Verification items for the finished model (mm, model axes). A direction names the side the tool comes from. Give positions to 0.01 mm unless a question says otherwise; leave off trailing zeros. Write each loop counter-clockwise with the first axis right and the second up, starting at its lowest first coordinate (ties: lowest second). Pieces come first, ordered by that corner, then holes. Notation, with made-up numbers: (25, 81.5) -> (32, 81.5) arc R25 cw to (32, 97.5) -> close; hole circle Ø7 at (21, 72). An arc over 180 degrees is marked (long way). Answer as CSV lines item,"result". Start each with the question number.
1) Tool access check on faces 4 (the flat face through (43, 3, 7)), 5 (the flat face through (14, 12, 11)), 6 (the flat face through (50, 3, 3)), 7 (the flat face through (7, 14, 21)). Record the directions out of +Z, -Z, +X, -X, +Y, -Y that give a thin tool (end or side, any length) a straight path to the whole face; none if there is none.
2) Mould release check, pull along Z, two halves, no side actions. Record for faces 1 (the flat face through (19, 0, 14)), 2 (the flat face through (43, 3, 21)), 3 (the flat face through (19, 6, 28)): released by +Z, released by -Z, zero draft, split by the parting line, or undercut.
3) Material ranges on L1, parallel to Y at x = 19, z = 7.75; L2, parallel to Y at x = 7.5, z = 16.5, recorded low to high.
4) Sectioned sample at A-A on y = 4.75. Record the cut outline in (x, z).
5) Sectioned sample at C-C on x = 5. Record the cut outline in (y, z), and give its area (3 significant figures).
6) Gauge pin test, flat ends, axial feed: pin 1 Ø4 at (x, z) = (10.5, 22.5) entering from +Y; pin 2 Ø4 at (x, y) = (19, 9.5) entering from +Z; pin 3 Ø14 at (x, z) = (35, 8) entering from +Y; pin 4 Ø3.5 at (x, y) = (6.5, 18.5) entering from +Z. Record the tip position at first contact, or that the pin passes through.
7) Sectioned sample at B-B on z = 24.5. Record the cut outline in (x, y).
8) Sectioned sample at D-D on y = 10. Record the cut outline in (x, z).
```python
from build123d import *

# Parameters (mm, degrees)
EXTRUDE_1_DEPTH     = 28
SKETCH_2_W          = 14
SKETCH_2_H          = 14
CUT_EXTRUDE_1_DEPTH = 7
CUT_EXTRUDE_2_REACH = 23


with BuildPart() as part:
    # 스케치1 → 보스-돌출1 (new body)
    with BuildSketch(Plane.XY):
        Polygon((14, 7), (14, 21), (0, 21), (0, 0), (50, 0), (50, 7), align=None)
    extrude(amount=EXTRUDE_1_DEPTH)

    # 스케치2 → 컷-돌출1 (cut)
    with BuildSketch(Plane(origin=(0, 21, 0), x_dir=(1, 0, 0), z_dir=(0, 1, 0))):
        with Locations((7, -21)):
            Rectangle(SKETCH_2_W, SKETCH_2_H)
    extrude(amount=-CUT_EXTRUDE_1_DEPTH, mode=Mode.SUBTRACT)

    # 스케치3 → 컷-돌출2 (cut, up to next)
    with BuildSketch(Plane(origin=(0, 0, 0), x_dir=(1, 0, 0), z_dir=(0, 1, 0)), mode=Mode.PRIVATE) as cut_extrude_2_sk1:
        with BuildLine():
            Line((36, -7), (50, -7))
            Line((50, -7), (50, -21))
            Line((50, -21), (36, -21))
            ThreePointArc((36, -21), (29, -14), (36, -7))
        make_face()
    cut_extrude_2_tool1 = extrude(cut_extrude_2_sk1.sketch, amount=CUT_EXTRUDE_2_REACH, mode=Mode.PRIVATE) & part.part
    add(cut_extrude_2_tool1.solids().sort_by_distance((40.188509, 0, 14))[0], mode=Mode.SUBTRACT)


solid = part.part
```
Ans:
1,face 4,"+X, +Y, -Y"
1,face 5,"+Z, -Z, +X, +Y"
1,face 6,"+Z, -Z, +X, +Y, -Y"
1,face 7,"+Z, +X, -X, +Y"
2,face 1,"zero draft"
2,face 2,"undercut"
2,face 3,"released by +Z"
3,L1,"y = 0 to 7"
3,L2,"y = 0 to 14"
4,outline,"(0, 0) -> (50, 0) -> (50, 7) -> (36, 7) arc R7 cw to (36, 21) -> (50, 21) -> (50, 28) -> (0, 28) -> close"
5,outline,"(0, 0) -> (21, 0) -> (21, 14) -> (14, 14) -> (14, 28) -> (0, 28) -> close"
5,area,"490 mm²"
6,pin 1,"stops at y = 14"
6,pin 2,"passes through"
6,pin 3,"stops at y = 7"
6,pin 4,"stops at z = 14"
7,outline,"(0, 0) -> (50, 0) -> (50, 7) -> (14, 7) -> (14, 14) -> (0, 14) -> close"
8,outline,"(0, 0) -> (14, 0) -> (14, 28) -> (0, 28) -> close"
